from build123d import *

# Parameters (mm, degrees)
SKETCH1_R               = 7.5
BOSS_EXTRUDE1_DEPTH     = 10
SKETCH2_R               = 4
BOSS_EXTRUDE2_DEPTH     = 15
SKETCH3_R               = 5
BOSS_EXTRUDE3_DEPTH     = 13
CUT_EXTRUDE1_DEPTH      = 40.452503089
CUT_EXTRUDE1_DEPTH_BACK = 7


with BuildPart() as part:
    # Sketch1 → Boss-Extrude1 (new body)
    with BuildSketch(Plane.XY):
        Circle(SKETCH1_R)
    extrude(amount=BOSS_EXTRUDE1_DEPTH)

    # Sketch2 → Boss-Extrude2 (add)
    with BuildSketch(Plane(origin=(0, 0, 0), x_dir=(-1, 0, 0), z_dir=(0, 0, -1))):
        Circle(SKETCH2_R)
    extrude(amount=BOSS_EXTRUDE2_DEPTH)

    # Sketch3 → Boss-Extrude3 (add)
    with BuildSketch(Plane(origin=(0, 0, -15), x_dir=(-1, 0, 0), z_dir=(0, 0, -1))):
        with Locations(Location((0, 0, 0), (0, 0, 180))):
            Circle(SKETCH3_R)
    extrude(amount=BOSS_EXTRUDE3_DEPTH)

    # Sketch4 → Cut-Extrude1 (cut, two sides: drawn at the far end of the back side and taken through both)
    with BuildSketch(Plane.XY.offset(10).offset(-CUT_EXTRUDE1_DEPTH_BACK)):
        Polygon((5.773502692, 0), (2.886751346, 5), (-2.886751346, 5), (-5.773502692, 0), (-2.886751346, -5), (2.886751346, -5), align=None)
    extrude(amount=CUT_EXTRUDE1_DEPTH + CUT_EXTRUDE1_DEPTH_BACK, mode=Mode.SUBTRACT)


solid = part.part
Can you work these out from the model? Positions are in its coordinate system, mm. A direction names the side the tool comes from. Round coordinates to 2 decimals unless told otherwise and drop trailing zeros. Loops run counter-clockwise (first coordinate to the right, second up) from the corner with the lowest first, then second, coordinate; pieces in that order, holes last. Notation, with made-up numbers: (39.5, 73.25) - (61.5, 73.25) arc R20 ccw to (61.5, 88.25) - close; hole circle Ø7 at (41, 13). An arc over 180 degrees is marked (long way). Write item = value, one per line. Start each with the question number.
(1) If we section it at A-A (z = 7): Please give me the cut outline in (x, y), and give its area (3 significant figures).
(2) If we section it at B-B (x = 0): Please give me the cut outline in (y, z).
(3) For P1, Ø2, axis at y = -1, z = -10, coming from the +X side; P2, Ø3, axis at x = -0.5, z = -9, coming from the +Y side; P3, Ø3, axis at x = 3, y = 6, coming from the -Z side, each with a flat end and sliding along its axis, tell me the tip position at first contact or that it passes through.
(4) If we section it at C-C (z = -9): Please give me the cut outline in (x, y), and give its area (3 significant figures).
(5) If we section it at D-D (y = -2): Please give me the cut outline in (x, z), and give its area (3 significant figures).
(6) For faces 4 (the face through (-5, 0, -21)), 5 (the face through (5, 2, 10)), 6 (the face through (-7.493, 0.33, 4.93)), 7 (the face through (4.31, -2.535, 6.451)), 8 (the face through (3, -3, 0)), which set-ups out of +Z, -Z, +X, -X, +Y, -Y let a thin tool reach every point of the face, with its end or its side?
(7) If we mould it in two halves opening along Y, with no side actions, what happens to faces 1 (the face through (4.35, 2.465, 6.451)), 2 (the face through (0, 0, -28)), 3 (the face through (0.867, -3.905, -7.395))? For each: released by +Y, released by -Y, zero draft, split by the parting line, or undercut.
(8) If I drill on probe 1 along Z at (x, y) = (2, -3.75); probe 2 along Y at (x, z) = (0.25, -17.5); probe 3 along Z at (x, y) = (-4, 5.75), over which ranges is the centre line in solid material (lowest first)? Write a range as [from, to].
Ans:
q1.outline = circle Ø15 at (0, 0); hole (-5.77, 0) - (-2.89, -5) - (2.89, -5) - (5.77, 0) - (2.89, 5) - (-2.89, 5) - close
q1.area = 90.1 mm²
q2.outline = (-7.5, 0) - (-4, 0) - (-4, -15) - (-5, -15) - (-5, -28) - (5, -28) - (5, -15) - (4, -15) - (4, 0) - (7.5, 0) - (7.5, 10) - (5, 10) - (5, 3) - (-5, 3) - (-5, 10) - (-7.5, 10) - close
q3.P1 = 4
q3.P2 = 4
q3.P3 = 0
q4.outline = circle Ø8 at (0, 0)
q4.area = 50.3 mm²
q5.outline = (-7.23, 0) - (-3.46, 0) - (-3.46, -15) - (-4.58, -15) - (-4.58, -28) - (4.58, -28) - (4.58, -15) - (3.46, -15) - (3.46, 0) - (7.23, 0) - (7.23, 10) - (4.62, 10) - (4.62, 3) - (-4.62, 3) - (-4.62, 10) - (-7.23, 10) - close
q5.area = 303 mm²
q6.face_4 = -Z
q6.face_5 = +Z, +X, -X, +Y, -Y
q6.face_6 = +Z, -Z
q6.face_7 = +Z
q6.face_8 = none
q7.face_1 = undercut
q7.face_2 = zero draft
q7.face_3 = split by the parting line
q8.probe_1 = [-28, -15], [0, 3]
q8.probe_2 = [-4.99, 4.99]
q8.probe_3 = [0, 10]
